```python
from build123d import *

# Parameters (mm, degrees)
F0_R     = 15.5
F0_R_2   = 12.5
F1_DEPTH = 15
F0_R_3   = 26
F0_R_4   = 22.5
F3_R     = 5
F4_DEPTH = 11


with BuildPart() as f1:
    # F0 (on Front) → F1 (new body)
    with BuildSketch(Plane.XZ):
        Circle(F0_R)
        Circle(F0_R_2, mode=Mode.SUBTRACT)
    extrude(amount=F1_DEPTH)



with BuildPart() as f1b:
    # F0 (on Front) → F1, piece 2 (new body)
    with BuildSketch(Plane.XZ):
        Circle(F0_R_3)
        Circle(F0_R_4, mode=Mode.SUBTRACT)
    extrude(amount=F1_DEPTH)


with BuildPart() as f1_1:
    add(f1.part)

    add(f1b.part)  # F4 merges F1b
    # F3 (on offset) → F4 (join)
    with BuildSketch(Plane.XZ):
        with Locations((0, 19)):
            Circle(F3_R)
        with Locations((11.1679197936, 15.3713228931)):
            Circle(F3_R)
        with Locations((18.0700738096, 5.8713228931)):
            Circle(F3_R)
        with Locations((18.0700738096, -5.8713228931)):
            Circle(F3_R)
        with Locations((11.1679197936, -15.3713228931)):
            Circle(F3_R)
        with Locations((0, -19)):
            Circle(F3_R)
        with Locations((-11.1679197936, -15.3713228931)):
            Circle(F3_R)
        with Locations((-18.0700738096, -5.8713228931)):
            Circle(F3_R)
        with Locations((-18.0700738096, 5.8713228931)):
            Circle(F3_R)
        with Locations((-11.1679197936, 15.3713228931)):
            Circle(F3_R)
    extrude(amount=F4_DEPTH)


solid = f1_1.part
```
Verification items for the finished model (mm, model axes). A direction names the side the tool comes from. Give positions to 0.01 mm unless a question says otherwise; leave off trailing zeros. Order: outer loops, then holes, each group sorted by start corner. A loop starts at its lowest first (then second) coordinate and runs counter-clockwise, first axis right, second up. Notation, with made-up numbers: (30, -31) - (55, -31) arc R28 ccw to (55, -7) - close; hole circle Ø1 at (83.5, 56). An arc over 180 degrees is marked (long way). Answer as CSV lines item,"result". Start each with the question number.
Item 1: Access from +Z, -Z, +X, -X, +Y, -Y to the whole of each face (thin tool, end or side, straight path). Record for faces 3 (the face through (18, -11, 6)), 4 (the face through (11.2, 0, 6.1)).
Item 2: Section check C-C, the plane y = -14. Record the boundary of the cut face in (x, z).
Item 3: Material ranges on L1, parallel to X at y = -5.75, z = -0.5; L2, parallel to Z at x = 0, y = -5; L3, parallel to Z at x = -3.5, y = -10, recorded low to high.
Item 4: Section check D-D, the plane z = -21. Record the boundary of the cut face in (x, y).
Item 5: Mould release check, pull along Z, two halves, no side actions. Record for faces 1 (the face through (-11.7, -15, 19.4)), 2 (the face through (-4.97, -5.42, -18.47)): released by +Z, released by -Z, zero draft, split by the parting line, or undercut.
Item 6: Gauge pin test, flat ends, axial feed: pin 1 (1 mm diameter, centred on y = -6.5, z = 9.5, fed in from +X); pin 2 (1.5 mm diameter, centred on x = 9.5, y = -12.5, fed in from -Z); pin 3 (1.5 mm diameter, centred on y = -2.5, z = -18, fed in from +X); pin 4 (15 mm diameter, centred on x = 0, z = 0, fed in from +Y). Record the tip position at first contact, or that the pin passes through.
Item 7: Section check A-A, the plane x = 0. Record the boundary of the cut face in (y, z), plus the area to 3 significant figures.
Item 8: Section check B-B, the plane z = 0. Record the boundary of the cut face in (x, y), plus the area to 3 significant figures.
Filled in:
1,face 3,"-Y"
1,face 4,"+Z, -Z, +X, -X, +Y"
2,outline,"circle Ø52 at (0, 0); circle Ø31 at (0, 0); hole circle Ø45 at (0, 0); hole circle Ø25 at (0, 0)"
3,L1,"-26 to -22.49, -15.49 to -12.49, 12.49 to 15.49, 22.49 to 26"
3,L2,"-26 to -12.5, 12.5 to 26"
3,L3,"-25.76 to -15.43, -15.1 to -12, 12 to 15.1, 15.43 to 25.76"
4,outline,"(-15.33, -15) - (-8.08, -15) - (-8.08, 0) - (-15.33, 0) - close; (-4.58, -11) - (4.58, -11) - (4.58, 0) - (-4.58, 0) - close; (8.08, -15) - (15.33, -15) - (15.33, 0) - (8.08, 0) - close"
5,face 1,"zero draft"
5,face 2,"undercut"
6,pin 1,"x = 24.39"
6,pin 2,"z = -24.48"
6,pin 3,"x = 19.45"
6,pin 4,"through"
7,outline,"(-15, -26) - (0, -26) - (0, -12.5) - (-15, -12.5) - (-15, -15.5) - (-11, -15.5) - (-11, -22.5) - (-15, -22.5) - close; (-15, 12.5) - (0, 12.5) - (0, 26) - (-15, 26) - (-15, 22.5) - (-11, 22.5) - (-11, 15.5) - (-15, 15.5) - close"
7,area,"349 mm^2"
8,outline,"(-26, -15) - (-22.5, -15) - (-22.5, 0) - (-26, 0) - close; (-15.5, -15) - (-12.5, -15) - (-12.5, 0) - (-15.5, 0) - close; (12.5, -15) - (15.5, -15) - (15.5, 0) - (12.5, 0) - close; (22.5, -15) - (26, -15) - (26, 0) - (22.5, 0) - close"
8,area,"195 mm^2"
